Part model, mm, in its own coordinate system. A direction names the side the tool comes from. Give positions to 0.01 mm unless a question says otherwise; leave off trailing zeros. Order: outer loops, then holes, each group sorted by start corner. A loop starts at its lowest first (then second) coordinate and runs counter-clockwise, first axis right, second up. Notation, with made-up numbers: M -28,-20 L 21,-20 A32 ccw 21,8 Z; hole C -13,-36 d1. An arc over 180 degrees is marked long. One line per question, with ' | ' between items.
```python
from build123d import *

# Parameters (mm, degrees)
SKETCH_1_W          = 53
SKETCH_1_H          = 44
SKETCH_1_W_2        = 84
SKETCH_1_H_2        = 35
EXTRUDE_1_DEPTH     = 5
SKETCH_2_R          = 1.6
CUT_EXTRUDE_1_DEPTH = 228.070473642


with BuildPart() as part:
    # 草图1 → 凸台-拉伸1 (new body)
    with BuildSketch(Plane.XY):
        Polygon((161, 0), (220, 0), (220, 56), (0, 56), (0, 0), (59, 0), (59, -30), (68, -30), (68, 9), (152, 9), (152, -30), (161, -30), align=None)
        with Locations((32.5, 28)):
            Rectangle(SKETCH_1_W, SKETCH_1_H, mode=Mode.SUBTRACT)
        with Locations((187.5, 28)):
            Rectangle(SKETCH_1_W, SKETCH_1_H, mode=Mode.SUBTRACT)
        with Locations((110, 32.5)):
            Rectangle(SKETCH_1_W_2, SKETCH_1_H_2, mode=Mode.SUBTRACT)
    extrude(amount=EXTRUDE_1_DEPTH)

    # 草图2 → 切除-拉伸1 (cut, through all)
    with BuildSketch(Plane.XY.offset(5)):
        with Locations((63, -15)):
            Circle(SKETCH_2_R)
        with Locations((157, -15)):
            Circle(SKETCH_2_R)
    extrude(amount=-CUT_EXTRUDE_1_DEPTH, mode=Mode.SUBTRACT)


solid = part.part
```
1. Slice it at B-B on z = 0.9. Give the cut face in (x, y), then the cut area to 3 significant figures.
Worked out:
outline: M 0,0 L 59,0 L 59,-30 L 68,-30 L 68,9 L 152,9 L 152,-30 L 161,-30 L 161,0 L 220,0 L 220,56 L 0,56 Z; hole M 6,6 L 59,6 L 59,50 L 6,50 Z; hole C 63,-15 d3.2; hole M 68,15 L 152,15 L 152,50 L 68,50 Z; hole C 157,-15 d3.2; hole M 161,6 L 214,6 L 214,50 L 161,50 Z | area: 4,480 mm2
2. Drop flat-ended pins along their axis: pin 1 (2.5 mm diameter, centred on y = -20, z = 3, fed in from -X); pin 2 (1.5 mm diameter, centred on x = 176.5, z = 3.5, fed in from -Y); pin 3 (2 mm diameter, centred on x = 120, y = 16.5, fed in from -Z); pin 4 (3 mm diameter, centred on y = -16.5, z = 2.5, fed in from +X). Give the stop position or say it passes through.
Worked out:
pin 1: stops at x = 59 | pin 2: stops at y = 0 | pin 3: passes through | pin 4: stops at x = 161
3. Probe L1, parallel to X at y = 41.5, z = 0.9; L2, parallel to Y at x = 172, z = 0.45; L3, parallel to Y at x = 63, z = 1.4. List the from-to ranges inside material, lowest first. Write a range as from..to.
Worked out:
L1: x = 0..6, 59..68, 152..161, 214..220 | L2: y = 0..6, 50..56 | L3: y = -30..-16.6, -13.4..56
4. Mould opens along Y. For faces 1 (the flat face through (29, 0, 2)), 2 (the flat face through (152, -10, 2)), 3 (the flat face through (152, 32, 2)) say: released by +Y, released by -Y, zero draft, split by the parting line, or undercut.
Worked out:
face 1: released by -Y | face 2: zero draft | face 3: undercut
5. Slice it at A-A on x = 41. Give the cut face in (y, z).
Worked out:
outline: M 0,0 L 6,0 L 6,5 L 0,5 Z; M 50,0 L 56,0 L 56,5 L 50,5 Z
6. Slice it at C-C on y = 39.5. Give the cut face in (x, z).
Worked out:
outline: M 0,0 L 6,0 L 6,5 L 0,5 Z; M 59,0 L 68,0 L 68,5 L 59,5 Z; M 152,0 L 161,0 L 161,5 L 152,5 Z; M 214,0 L 220,0 L 220,5 L 214,5 Z
7. Tool access for faces 4 (the flat face through (63, -30, 2)), 5 (the flat face through (109, 9, 2)), 6 (the flat face through (161, -15, 2)), 7 (the flat face through (6, 28, 2)): list every direction of +Z, -Z, +X, -X, +Y, -Y with a clear straight run to the whole face (end or side of a thin tool).
Worked out:
face 4: +Z, -Z, +X, -X, -Y | face 5: +Z, -Z, -Y | face 6: +Z, -Z, +X, -Y | face 7: +Z, -Z
